```python
from build123d import *

# Parameters (mm, degrees)
CROQUIS1_W              = 17
CROQUIS1_H              = 7
SALIENTE_EXTRUIR1_DEPTH = 7
CROQUIS2_R              = 2.51
CROQUIS2_W              = 7.1
CROQUIS2_H              = 5.1
CORTAR_EXTRUIR2_DEPTH   = 7
CROQUIS4_W              = 0.7
CROQUIS4_H              = 0.6
CORTAR_EXTRUIR3_DEPTH   = 2
CROQUIS5_W              = 0.5
CROQUIS5_H              = 0.344672938
CROQUIS5_H_2            = 0.308474041
CORTAR_EXTRUIR4_DEPTH   = 2


with BuildPart() as part:
    # Croquis1 → Saliente-Extruir1 (new body)
    with BuildSketch(Plane.XY):
        with Locations((5.190566528, 3.234615385)):
            Rectangle(CROQUIS1_W, CROQUIS1_H)
    extrude(amount=SALIENTE_EXTRUIR1_DEPTH)

    # Croquis2 → Cortar-Extruir2 (cut)
    with BuildSketch(Plane(origin=(0, 0, 0), x_dir=(-1, 0, 0), z_dir=(0, 0, -1))):
        with Locations((-0.940566528, 3.234615385)):
            Circle(CROQUIS2_R)
        with Locations((-9.440566528, 3.234615385)):
            Rectangle(CROQUIS2_W, CROQUIS2_H)
    extrude(amount=-CORTAR_EXTRUIR2_DEPTH, mode=Mode.SUBTRACT)

    # Croquis4 → Cortar-Extruir3 (cut)
    with BuildSketch(Plane(origin=(0, 0, 0), x_dir=(-1, 0, 0), z_dir=(0, 0, -1))):
        with Locations((-13.340566528, 5.829288323)):
            Rectangle(CROQUIS4_W, CROQUIS4_H)
        with Locations((-13.340566528, 3.346068945)):
            Rectangle(CROQUIS4_W, CROQUIS4_H)
        with Locations((-13.340566528, 0.676141344)):
            Rectangle(CROQUIS4_W, CROQUIS4_H)
    extrude(amount=-CORTAR_EXTRUIR3_DEPTH, mode=Mode.SUBTRACT)

    # Croquis5 → Cortar-Extruir4 (cut)
    with BuildSketch(Plane(origin=(0, 0, 0), x_dir=(-1, 0, 0), z_dir=(0, 0, -1))):
        with Locations((-12.740566528, 5.956951854)):
            Rectangle(CROQUIS5_W, CROQUIS5_H)
        with Locations((-12.740566528, 0.530378365)):
            Rectangle(CROQUIS5_W, CROQUIS5_H_2)
    extrude(amount=-CORTAR_EXTRUIR4_DEPTH, mode=Mode.SUBTRACT)


solid = part.part
```
Here's how the part is built. I have some questions about the finished solid (model axes, mm). A direction names the side the tool comes from. Coordinates: 2 decimals unless noted, no trailing zeros. Order: outer loops, then holes, each group sorted by start corner. A loop starts at its lowest first (then second) coordinate and runs counter-clockwise, first axis right, second up.
1) Which directions (+Z, -Z, +X, -X, +Y, -Y) give clear straight access to the entire face, cutting with the end or side of a thin tool? Please do faces 1 (the face through (3, 5, 0)), 2 (the face through (5.891, 3, 3)), 3 (the face through (13, 6.129, 1)).
2) Will this pin go through, and if not, where does the flat tip stop? pin 1 (1.5 mm diameter, centred on x = 9, y = 4, fed in from -Z).
3) Imagine slicing it at D-D on z = 4. List the corners of the cut face in (x, y) for me, and give its area (3 significant figures).
4) We'd pull the mould along X, two halves only. Please class faces 4 (the face through (9, 5.785, 3)), 5 (the face through (13.691, 3, 3)), 6 (the face through (13, 0.376, 1)): +X half, -X half, draft (parallel to the pull), parting line (faces both ways), or undercut.
5) Imagine slicing it at C-C on z = 0.75. List the corners of the cut face in (x, y) for me, and give its area (3 significant figures).
6) I need wall thicknesses on line 1 (Y direction, x = 6, z = 4.75); line 2 (X direction, y = 5.25, z = 3.5); line 3 (X direction, y = 5.5, z = 6.25). Which ranges of each line are inside material? Lowest first, please.
7) Imagine slicing it at B-B on y = 4.5. List the corners of the cut face in (x, z) for me, and give its area (3 significant figures).
8) Imagine slicing it at A-A on x = 8.5. List the corners of the cut face in (y, z) for me.
Response values:
1. face 1: -Z, +X, -X, +Y, -Y
1. face 2: +Z, -Z
1. face 3: -Z, +X
2. pin 1: passes through
3. outline: (-3.31, -0.27) - (13.69, -0.27) - (13.69, 6.73) - (-3.31, 6.73) - close; hole circle Ø5.02 at (0.94, 3.23); hole (5.89, 0.68) - (12.99, 0.68) - (12.99, 5.78) - (5.89, 5.78) - close
3. area: 63.0 mm2
4. face 4: undercut
4. face 5: +X half
4. face 6: draft
5. outline: (-3.31, -0.27) - (13.69, -0.27) - (13.69, 0.38) - (12.49, 0.38) - (12.49, 0.68) - (5.89, 0.68) - (5.89, 5.78) - (12.49, 5.78) - (12.49, 6.13) - (13.69, 6.13) - (13.69, 6.73) - (-3.31, 6.73) - close; (12.99, 0.98) - (13.69, 0.98) - (13.69, 3.05) - (12.99, 3.05) - close; (12.99, 3.65) - (13.69, 3.65) - (13.69, 5.53) - (12.99, 5.53) - close; hole circle Ø5.02 at (0.94, 3.23)
5. area: 61.4 mm2
6. line 1: y = -0.27 to 0.68, 5.78 to 6.73
6. line 2: x = -3.31 to -0.56, 2.44 to 5.89, 12.99 to 13.69
6. line 3: x = -3.31 to -0.14, 2.02 to 5.89, 12.99 to 13.69
7. outline: (-3.31, 0) - (-1.23, 0) - (-1.23, 7) - (-3.31, 7) - close; (3.11, 0) - (5.89, 0) - (5.89, 7) - (3.11, 7) - close; (12.99, 0) - (13.69, 0) - (13.69, 7) - (12.99, 7) - close
7. area: 39.0 mm2
8. outline: (-0.27, 0) - (0.68, 0) - (0.68, 7) - (-0.27, 7) - close; (5.78, 0) - (6.73, 0) - (6.73, 7) - (5.78, 7) - close
